from build123d import *

# Parameters (mm, degrees)
SKETCH_1_W             = 610
SKETCH_1_H             = 420
EXTRUDE_1_DEPTH        = 6
HOLE_WIZARD_M6_1_D     = 5
HOLE_WIZARD_M6_1_DEPTH = 15
HOLE_WIZARD_M6_1_TIP   = 1.502151548
HOLE_WIZARD_M5_1_D     = 4.2
HOLE_WIZARD_M5_1_DEPTH = 12.4
HOLE_WIZARD_M5_1_TIP   = 1.2618073
HOLE_WIZARD_M5_2_D     = 4.2
HOLE_WIZARD_M5_2_DEPTH = 12.4
HOLE_WIZARD_M5_2_TIP   = 1.2618073
HOLE_WIZARD_M6_2_D     = 5
HOLE_WIZARD_M6_2_DEPTH = 15
HOLE_WIZARD_M6_2_TIP   = 1.502151548
HOLE_WIZARD_M5_3_D     = 4.2
HOLE_WIZARD_M5_3_DEPTH = 12.4
HOLE_WIZARD_M5_3_TIP   = 1.2618073
HOLE_WIZARD_M5_4_D     = 4.2
HOLE_WIZARD_M5_4_DEPTH = 12.4
HOLE_WIZARD_M5_4_TIP   = 1.2618073
HOLE_WIZARD_M5_5_D     = 4.2
HOLE_WIZARD_M5_5_DEPTH = 12.4
HOLE_WIZARD_M5_5_TIP   = 1.2618073
HOLE_WIZARD_M5_6_D     = 4.2
HOLE_WIZARD_M5_6_DEPTH = 12.4
HOLE_WIZARD_M5_6_TIP   = 1.2618073
HOLE_WIZARD_M5_7_D     = 4.2
HOLE_WIZARD_M5_7_DEPTH = 12.4
HOLE_WIZARD_M5_7_TIP   = 1.2618073
SKETCH_22_W            = 610
SKETCH_22_H            = 6
EXTRUDE_2_DEPTH        = 47.17
SKETCH_23_W            = 610
SKETCH_23_H            = 6
EXTRUDE_3_DEPTH        = 90
SKETCH_24_W            = 6
SKETCH_24_H            = 557.17
EXTRUDE_4_DEPTH        = 39.94
SKETCH_25_W            = 6
SKETCH_25_H            = 557.17
EXTRUDE_5_DEPTH        = 100.06
SKETCH_26_W            = 250
SKETCH_26_H            = 110
CUT_EXTRUDE_1_DEPTH    = 100.06
CHAMFER_2_SIZE         = 2
CHAMFER_3_SIZE         = 2
CHAMFER_4_SIZE         = 2
CHAMFER_5_SIZE         = 2
HOLE_WIZARD_M4_1_D     = 3.3
HOLE_WIZARD_M4_1_DEPTH = 10.1
HOLE_WIZARD_M4_1_TIP   = 0.991420021
HOLE_WIZARD_M4_2_D     = 3.3
HOLE_WIZARD_M4_2_DEPTH = 10.1
HOLE_WIZARD_M4_2_TIP   = 0.991420021
HOLE_WIZARD_M4_3_D     = 3.3
HOLE_WIZARD_M4_3_DEPTH = 10.1
HOLE_WIZARD_M4_3_TIP   = 0.991420021
HOLE_WIZARD_M4_4_D     = 3.3
HOLE_WIZARD_M4_4_DEPTH = 10.1
HOLE_WIZARD_M4_4_TIP   = 0.991420021
HOLE_WIZARD_M4_5_D     = 3.3
HOLE_WIZARD_M4_5_DEPTH = 10.1
HOLE_WIZARD_M4_5_TIP   = 0.991420021


with BuildPart() as part:
    # 草图1 → 凸台-拉伸1 (new body)
    with BuildSketch(Plane.XY):
        with Locations((305, 210)):
            Rectangle(SKETCH_1_W, SKETCH_1_H)
    extrude(amount=EXTRUDE_1_DEPTH)

    # M6 螺纹孔1
    with Locations(Plane.XY.offset(6)):
        with Locations((99, 410.6), (139, 410.6)):
            Hole(HOLE_WIZARD_M6_1_D / 2, depth=HOLE_WIZARD_M6_1_DEPTH)
            with Locations((0, 0, -(HOLE_WIZARD_M6_1_DEPTH + HOLE_WIZARD_M6_1_TIP / 2))):  # 118° drill point
                Cone(0, HOLE_WIZARD_M6_1_D / 2, HOLE_WIZARD_M6_1_TIP, mode=Mode.SUBTRACT)

    # M5 螺纹孔1
    with Locations(Plane.XY.offset(6)):
        with Locations((10.231581543, 318.9), (22.231581543, 318.9)):
            Hole(HOLE_WIZARD_M5_1_D / 2, depth=HOLE_WIZARD_M5_1_DEPTH)
            with Locations((0, 0, -(HOLE_WIZARD_M5_1_DEPTH + HOLE_WIZARD_M5_1_TIP / 2))):  # 118° drill point
                Cone(0, HOLE_WIZARD_M5_1_D / 2, HOLE_WIZARD_M5_1_TIP, mode=Mode.SUBTRACT)

    # M5 螺纹孔2
    with Locations(Plane.XY.offset(6)):
        with Locations((10.231581543, 210.9), (22.231581543, 210.9)):
            Hole(HOLE_WIZARD_M5_2_D / 2, depth=HOLE_WIZARD_M5_2_DEPTH)
            with Locations((0, 0, -(HOLE_WIZARD_M5_2_DEPTH + HOLE_WIZARD_M5_2_TIP / 2))):  # 118° drill point
                Cone(0, HOLE_WIZARD_M5_2_D / 2, HOLE_WIZARD_M5_2_TIP, mode=Mode.SUBTRACT)

    # M6 螺纹孔2
    with Locations(Plane.XY.offset(6)):
        with Locations((99, 109.6), (139, 109.6)):
            Hole(HOLE_WIZARD_M6_2_D / 2, depth=HOLE_WIZARD_M6_2_DEPTH)
            with Locations((0, 0, -(HOLE_WIZARD_M6_2_DEPTH + HOLE_WIZARD_M6_2_TIP / 2))):  # 118° drill point
                Cone(0, HOLE_WIZARD_M6_2_D / 2, HOLE_WIZARD_M6_2_TIP, mode=Mode.SUBTRACT)

    # M5 螺纹孔3
    with Locations(Plane.XY.offset(6)):
        with Locations((515, 367.9), (515, 327.9), (605, 327.9), (605, 367.9)):
            Hole(HOLE_WIZARD_M5_3_D / 2, depth=HOLE_WIZARD_M5_3_DEPTH)
            with Locations((0, 0, -(HOLE_WIZARD_M5_3_DEPTH + HOLE_WIZARD_M5_3_TIP / 2))):  # 118° drill point
                Cone(0, HOLE_WIZARD_M5_3_D / 2, HOLE_WIZARD_M5_3_TIP, mode=Mode.SUBTRACT)

    # M5 螺纹孔4
    with Locations(Plane.XY.offset(6)):
        with Locations((582.231581543, 277.4), (594.231581543, 277.4), (509.3, 268.5), (509.3, 256.5), (509.3, 16), (509.3, 4), (577.3, 16), (577.3, 4), (577.3, 95), (577.3, 107)):
            Hole(HOLE_WIZARD_M5_4_D / 2, depth=HOLE_WIZARD_M5_4_DEPTH)
            with Locations((0, 0, -(HOLE_WIZARD_M5_4_DEPTH + HOLE_WIZARD_M5_4_TIP / 2))):  # 118° drill point
                Cone(0, HOLE_WIZARD_M5_4_D / 2, HOLE_WIZARD_M5_4_TIP, mode=Mode.SUBTRACT)

    # M5 螺纹孔5
    with Locations(Plane.XY.offset(6)):
        with Locations((220.520192359, 277.4), (232.520192359, 277.4)):
            Hole(HOLE_WIZARD_M5_5_D / 2, depth=HOLE_WIZARD_M5_5_DEPTH)
            with Locations((0, 0, -(HOLE_WIZARD_M5_5_DEPTH + HOLE_WIZARD_M5_5_TIP / 2))):  # 118° drill point
                Cone(0, HOLE_WIZARD_M5_5_D / 2, HOLE_WIZARD_M5_5_TIP, mode=Mode.SUBTRACT)

    # M5 螺纹孔6
    with Locations(Plane.XY.offset(6)):
        with Locations((324.3072517, 91.214749506), (389.3072517, 91.214749506)):
            Hole(HOLE_WIZARD_M5_6_D / 2, depth=HOLE_WIZARD_M5_6_DEPTH)
            with Locations((0, 0, -(HOLE_WIZARD_M5_6_DEPTH + HOLE_WIZARD_M5_6_TIP / 2))):  # 118° drill point
                Cone(0, HOLE_WIZARD_M5_6_D / 2, HOLE_WIZARD_M5_6_TIP, mode=Mode.SUBTRACT)

    # M5 螺纹孔7
    with Locations(Plane.XY.offset(6)):
        with Locations((324.3072517, 401.214749506), (389.3072517, 401.214749506)):
            Hole(HOLE_WIZARD_M5_7_D / 2, depth=HOLE_WIZARD_M5_7_DEPTH)
            with Locations((0, 0, -(HOLE_WIZARD_M5_7_DEPTH + HOLE_WIZARD_M5_7_TIP / 2))):  # 118° drill point
                Cone(0, HOLE_WIZARD_M5_7_D / 2, HOLE_WIZARD_M5_7_TIP, mode=Mode.SUBTRACT)

    # 草图22 → 凸台-拉伸2 (add)
    with BuildSketch(Plane.XZ):
        with Locations((305, 3)):
            Rectangle(SKETCH_22_W, SKETCH_22_H)
    extrude(amount=EXTRUDE_2_DEPTH)

    # 草图23 → 凸台-拉伸3 (add)
    with BuildSketch(Plane(origin=(0, 420, 0), x_dir=(1, 0, 0), z_dir=(0, 1, 0))):
        with Locations((305, -3)):
            Rectangle(SKETCH_23_W, SKETCH_23_H)
    extrude(amount=EXTRUDE_3_DEPTH)

    # 草图24 → 凸台-拉伸4 (add)
    with BuildSketch(Plane.ZY):
        with Locations((3, 231.415)):
            Rectangle(SKETCH_24_W, SKETCH_24_H)
    extrude(amount=EXTRUDE_4_DEPTH)

    # 草图25 → 凸台-拉伸5 (add)
    with BuildSketch(Plane(origin=(610, 0, 0), x_dir=(0, 0, -1), z_dir=(1, 0, 0))):
        with Locations((-3, 231.415)):
            Rectangle(SKETCH_25_W, SKETCH_25_H)
    extrude(amount=EXTRUDE_5_DEPTH)

    # 草图26 → 切除-拉伸1 (cut)
    with BuildSketch(Plane.XY.offset(6)):
        with Locations((585.06, 455)):
            Rectangle(SKETCH_26_W, SKETCH_26_H)
    extrude(amount=-CUT_EXTRUDE_1_DEPTH, mode=Mode.SUBTRACT)

    # 倒角2
    chamfer_2_edges = [part.edges().sort_by_distance(p)[0] for p in [
        (710.06, -47.17, 3),
    ]]
    chamfer(chamfer_2_edges, length=CHAMFER_2_SIZE)

    # 倒角3
    chamfer_3_edges = [part.edges().sort_by_distance(p)[0] for p in [
        (-39.94, -47.17, 3),
    ]]
    chamfer(chamfer_3_edges, length=CHAMFER_3_SIZE)

    # 倒角4
    chamfer_4_edges = [part.edges().sort_by_distance(p)[0] for p in [
        (-39.94, 510, 3),
    ]]
    chamfer(chamfer_4_edges, length=CHAMFER_4_SIZE)

    # 倒角5
    chamfer_5_edges = [part.edges().sort_by_distance(p)[0] for p in [
        (460.06, 510, 3),
    ]]
    chamfer(chamfer_5_edges, length=CHAMFER_5_SIZE)

    # M4 螺纹孔1
    with Locations(Plane(origin=(0, -47.17, 0), x_dir=(-1, 0, 0), z_dir=(0, -1, 0))):
        with Locations((-35.061581543, -3), (-135.061581543, -3), (-235.061581543, -3), (-435.061581543, -3), (-535.061581543, -3), (-635.061581543, -3)):
            Hole(HOLE_WIZARD_M4_1_D / 2, depth=HOLE_WIZARD_M4_1_DEPTH)
            with Locations((0, 0, -(HOLE_WIZARD_M4_1_DEPTH + HOLE_WIZARD_M4_1_TIP / 2))):  # 118° drill point
                Cone(0, HOLE_WIZARD_M4_1_D / 2, HOLE_WIZARD_M4_1_TIP, mode=Mode.SUBTRACT)

    # M4 螺纹孔2
    with Locations(Plane.ZY.offset(39.94)):
        with Locations((3, 471.4166), (3, 391.4166), (3, 311.4166), (3, 151.4166), (3, 71.4166), (3, -8.5834)):
            Hole(HOLE_WIZARD_M4_2_D / 2, depth=HOLE_WIZARD_M4_2_DEPTH)
            with Locations((0, 0, -(HOLE_WIZARD_M4_2_DEPTH + HOLE_WIZARD_M4_2_TIP / 2))):  # 118° drill point
                Cone(0, HOLE_WIZARD_M4_2_D / 2, HOLE_WIZARD_M4_2_TIP, mode=Mode.SUBTRACT)

    # M4 螺纹孔3
    with Locations(Plane(origin=(0, 510, 0), x_dir=(1, 0, 0), z_dir=(0, 1, 0))):
        with Locations((361.179881543, -3), (311.179881543, -3), (261.179881543, -3), (161.179881543, -3), (111.179881543, -3), (61.179881543, -3)):
            Hole(HOLE_WIZARD_M4_3_D / 2, depth=HOLE_WIZARD_M4_3_DEPTH)
            with Locations((0, 0, -(HOLE_WIZARD_M4_3_DEPTH + HOLE_WIZARD_M4_3_TIP / 2))):  # 118° drill point
                Cone(0, HOLE_WIZARD_M4_3_D / 2, HOLE_WIZARD_M4_3_TIP, mode=Mode.SUBTRACT)

    # M4 螺纹孔4
    with Locations(Plane(origin=(710.06, 0, 0), x_dir=(0, 0, -1), z_dir=(1, 0, 0))):
        with Locations((-3, -3.2184), (-3, 56.7816), (-3, 116.7816), (-3, 236.7816), (-3, 296.7816), (-3, 356.7816)):
            Hole(HOLE_WIZARD_M4_4_D / 2, depth=HOLE_WIZARD_M4_4_DEPTH)
            with Locations((0, 0, -(HOLE_WIZARD_M4_4_DEPTH + HOLE_WIZARD_M4_4_TIP / 2))):  # 118° drill point
                Cone(0, HOLE_WIZARD_M4_4_D / 2, HOLE_WIZARD_M4_4_TIP, mode=Mode.SUBTRACT)

    # M4 螺纹孔5
    with Locations(Plane(origin=(0, 400, 0), x_dir=(1, 0, 0), z_dir=(0, 1, 0))):
        with Locations((666.061581543, -3), (626.061581543, -3), (546.061581543, -3), (506.061581543, -3)):
            Hole(HOLE_WIZARD_M4_5_D / 2, depth=HOLE_WIZARD_M4_5_DEPTH)
            with Locations((0, 0, -(HOLE_WIZARD_M4_5_DEPTH + HOLE_WIZARD_M4_5_TIP / 2))):  # 118° drill point
                Cone(0, HOLE_WIZARD_M4_5_D / 2, HOLE_WIZARD_M4_5_TIP, mode=Mode.SUBTRACT)


solid = part.part
Source: CAD feature listing. Evaluate the final solid. Frame: model axes, mm. Coordinates: 2 decimals unless noted, no trailing zeros. Loops run counter-clockwise (first coordinate to the right, second up) from the corner with the lowest first, then second, coordinate; pieces in that order, holes last. Notation, with made-up numbers: (-27.5, -38.75) - (-8.5, -38.75) arc R25 cw to (-8.5, -3.75) - close; hole circle Ø5 at (12.5, 63.5). An arc over 180 degrees is marked (long way). Return JSON: item names as keys, results as strings.
Q1. Contact query for flat-ended pins moving along their axis: P1, Ø3.5, axis at x = 515, y = 327.9, coming from the +Z side; P2, Ø2.5, axis at x = 635.06, z = 3, coming from the +Y side; P3, Ø2, axis at y = 311.42, z = 3, coming from the -X side; P4, Ø3, axis at y = 296.78, z = 3, coming from the +X side. Output: stop coordinate, or through.
Results:
{"P1": "through", "P2": "y = 400", "P3": "x = -29.45", "P4": "x = 699.87"}
Q2. Material intervals for line 1 along X through (y, z) = (410.6, 2.25); line 2 along X through (y, z) = (394.5, 2.6); line 3 along X through (y, z) = (393, 2.3), sorted ascending.
Results:
{"line 1": "-39.94 to 96.5, 101.5 to 136.5, 141.5 to 460.06", "line 2": "-39.94 to 504.46, 507.66 to 544.46, 547.66 to 624.46, 627.66 to 664.46, 667.66 to 710.06", "line 3": "-39.94 to 504.57, 507.56 to 544.57, 547.56 to 624.57, 627.56 to 664.57, 667.56 to 710.06"}
Q3. Section A-A, the plane x = 655.5. Return loops of the section in (y, z).
Results:
{"outline": "(-47.17, 0) - (400, 0) - (400, 6) - (-47.17, 6) - close"}
